Autodesk Inventor part; units mm, degrees
ref_plane "YZ Plane" through (0, 0, 0) normal (1, 0, 0) x (0, 1, 0)
ref_plane "XZ Plane" through (0, 0, 0) normal (0, 1, 0) x (-1, 0, 0)
ref_plane "XY Plane" through (0, 0, 0) normal (0, 0, 1) x (1, 0, 0)
sketch "Sketch1" plane through (0, 0, 0) normal (0, 1, 0) x (-1, 0, 0)
  line L0 (0, 0) -> (9.899, 0)
  line L1 (9.899, 0) -> (9.899, -17.899)
  line L2 (9.899, -17.899) -> (0, -17.899)
  line L3 (0, -17.899) -> (0, 0)
  line L4 (0.5, -0.5) -> (9.399, -0.5)
  line L5 (9.399, -0.5) -> (9.399, -17.399)
  line L6 (9.399, -17.399) -> (0.5, -17.399)
  line L7 (0.5, -17.399) -> (0.5, -0.5)
  dimension "d0" = 9.899
  dimension "d1" = 17.899
  dimension "d2" = 16.899
  dimension "d3" = 8.899
  dimension "d4" = 0.5
  dimension "d5" = 0.5
sketch "Sketch3" plane through (0, 0, 0) normal (1, 0, 0) x (0, 1, 0)
  arc A0 (0, 0) -> (11.2583, 6.5) centre (0, 13) ccw
  line L0 (0, 13) -> (11.2583, 6.5) construction
  line L1 (0, 13) -> (0, 0) construction
  dimension "d6" = 60
  dimension "d7" = 13
sweep "Sweep1" add profiles "Sketch1" path "Sketch3"
extrude "Extrusion1" add sketch "Sketch1" against normal blind 16.55
ref_plane "Work Plane1" through (-9.899, 11.2583, 6.5) normal (0, 0.5, 0.866) x (1, 0, 0)
sketch "Sketch4" plane through (-9.899, 11.2583, 6.5) normal (0, 0.5, 0.866) x (1, 0, 0)
  line L0 (0, 0) -> (9.899, 0)
  line L1 (0, 0) -> (0, 17.899)
  line L2 (0, 17.899) -> (9.899, 17.899)
  line L3 (9.899, 17.899) -> (9.899, 0)
  line L4 (0.5, 17.399) -> (9.399, 17.399)
  line L5 (9.399, 17.399) -> (9.399, 0.5)
  line L6 (9.399, 0.5) -> (0.5, 0.5)
  line L7 (9.399, 0.5) -> (0.5, 0.5)
  line L8 (0.5, 0.5) -> (0.5, 17.399)
extrude "Extrusion2" add sketch "Sketch4" along normal blind 16.55
properties part number "curved waveguide120"
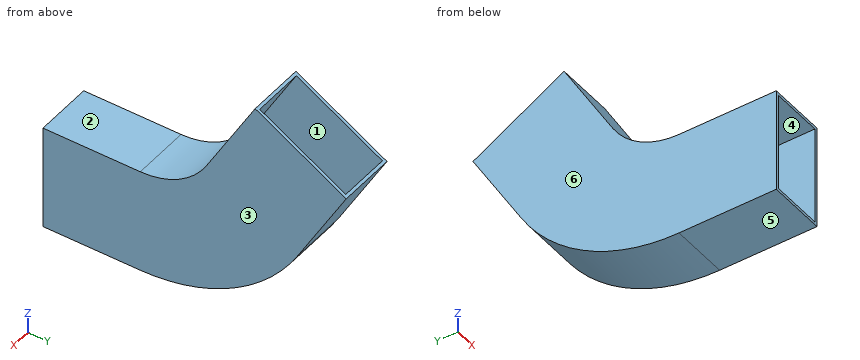
CAD build for the part. Positions are in the model's coordinates, mm. Face numbers are marked on the shaded views. A direction names the side the tool comes from. Round coordinates to 2 decimals unless told otherwise and drop trailing zeros. Loops run counter-clockwise (first coordinate to the right, second up) from the corner with the lowest first, then second, coordinate; pieces in that order, holes last. Notation, with made-up numbers: M -30,56 L 14,56 A12 cw 14,76 Z; hole C 89,72 d2. An arc over 180 degrees is marked long. Return JSON: item names as keys, results as strings. Group by question number.
(1) Saw through at C-C, the plane z = 10.5. List the corners of the cut face in (x, y), and give its area (3 significant figures).
(2) Wall check: probe 1 along X at (y, z) = (-7.5, -16); probe 2 along Z at (x, y) = (-2, -10.5); probe 3 along Z at (x, y) = (-2, 15). Give the ranges that are in metal, low to high. Write a range as [from, to].
(3) Saw through at A-A, the plane x = -3.75. List the corners of the cut face in (y, z), and give its area (3 significant figures).
(4) Saw through at D-D, the plane y = 29.5. List the corners of the cut face in (x, z).
(5) Tool access for the marked faces 1, 2 and 3: list every direction of +Z, -Z, +X, -X, +Y, -Y with a clear straight run to the whole face (end or side of a thin tool).
(6) Saw through at B-B, the plane y = -4. List the corners of the cut face in (x, z), and give its area (3 significant figures).
(7) Drop flat-ended pins along their axis: P1, Ø2, axis at x = -5, y = 26.5, coming from the -Z side; P2, Ø1.5, axis at x = -3.5, y = 18, coming from the +Z side; P3, Ø5, axis at y = 9.5, z = 10, coming from the +X side; P4, Ø1, axis at x = -6, z = 16, coming from the -Y side. Give the stop position or say it passes through.
(8) Mould opens along Z. For the marked faces 4, 5 and 6 say: +Z half, -Z half, draft (parallel to the pull), parting line (faces both ways), or undercut.
Answer list:
{
 "1": {"outline": "M -9.9,13.57 L 0,13.57 L 0,34.24 L -9.9,34.24 Z; hole M -9.4,14.15 L -0.5,14.15 L -0.5,33.66 L -9.4,33.66 Z", "area": "30.9 mm2"},
 "2": {"probe 1": "[-9.9, -9.4], [-0.5, 0]", "probe 2": "[-17.9, -17.4], [-0.5, 0]", "probe 3": "[-14.01, -13.44], [11.98, 12.98]"},
 "3": {"outline": "M -16.55,-17.9 L 0,-17.9 A30.9 ccw 26.76,-2.45 L 35.03,11.88 L 34.6,12.13 L 26.33,-2.2 A30.4 cw 0,-17.4 L -16.55,-17.4 Z; M -16.55,-0.5 L 0,-0.5 A13.5 ccw 11.69,6.25 L 19.97,20.58 L 19.53,20.83 L 11.26,6.5 A13 cw 0,0 L -16.55,0 Z", "area": "56.1 mm2"},
 "4": {"outline": "M -9.9,2.3 L 0,2.3 L 0,15.08 L -0.5,15.08 L -0.5,3.3 L -9.4,3.3 L -9.4,15.08 L -9.9,15.08 Z"},
 "5": {"face 1": "none", "face 2": "+Z, +X, -X, -Y", "face 3": "+Z, -Z, +X, +Y, -Y"},
 "6": {"outline": "M -9.9,-17.9 L 0,-17.9 L 0,0 L -9.9,0 Z; hole M -9.4,-17.4 L -0.5,-17.4 L -0.5,-0.5 L -9.4,-0.5 Z", "area": "26.8 mm2"},
 "7": {"P1": "z = -4.45", "P2": "z = 19.48", "P3": "through", "P4": "y = 16.45"},
 "8": {"face 4": "undercut", "face 5": "-Z half", "face 6": "draft"}
}
